Part model, mm, in its own coordinate system. A direction names the side the tool comes from. Coordinates: 2 decimals unless noted, no trailing zeros. Write each loop counter-clockwise with the first axis right and the second up, starting at its lowest first coordinate (ties: lowest second). Pieces come first, ordered by that corner, then holes. Notation, with made-up numbers: (61.25, 64.5) -> (89.25, 64.5) arc R15 cw to (89.25, 85.5) -> close; hole circle Ø9 at (44, 24.25). An arc over 180 degrees is marked (long way). One line per question, with ' | ' between items. Start each with the question number.
Item 1: Pin check, flat tips, straight feed: pin 1 (3.5 mm diameter, centred on x = 1.5, y = 0, fed in from -Z); pin 2 (4 mm diameter, centred on x = -12.5, y = 4, fed in from +Z); pin 3 (0.8 mm diameter, centred on x = 4, z = -1, fed in from +Y); pin 4 (2 mm diameter, centred on x = 7, z = 0.15, fed in from +Y). Stop position of each tip, or through.
Item 2: Saw through at D-D (z = 5). List the corners of the cut face in (x, y).
Item 3: Saw through at C-C (y = 0). Count the separate pieces of the cut face and the enclosed holes in it, and give its area (3 significant figures).
Item 4: Two-plate mould, pull along X, no slides. Class faces 1 (the flat face through (4, 1, -2)), 2 (the cylindrical face through (3, 0, 10)), 3 (the cylindrical face through (-17.32, -1.7, -11.74)), 4 (the cylindrical face through (5.29, 0.08, -0.23)): pulls with the +X half, pulls with the -X half, needs draft (parallel to the pull), parting line crosses it, or undercut.
Item 5: Probe probe 1 along Y at (x, z) = (-8, -6.35); probe 2 along Z at (x, y) = (3.5, 0.5); probe 3 along X at (y, z) = (-4, 1.25) (3 decimals). List the from-to ranges inside material, lowest first. Write a range as [from, to].
Item 6: Saw through at A-A (x = -7). List the corners of the cut face in (y, z), and give its area (3 significant figures).
Item 7: Saw through at B-B (x = 0). List the corners of the cut face in (y, z), and give its area (3 significant figures).
Item 8: 3-axis set-ups, long thin cutter, end or side, ignore diameter. For faces 5 (the cylindrical face through (7.751, -0.079, 2.535)), 6 (the cylindrical face through (-5.39, -1.7, 10.97)), 7 (the cylindrical face through (0, 2.5, -2)), 8 (the flat face through (4, -1, -2)): which of +Z, -Z, +X, -X, +Y, -Y reach the whole face in a straight line?
from build123d import *

# Parameters (mm, degrees)
BOSS_EXTRUDE1_DEPTH      = 5.65
BOSS_EXTRUDE1_DEPTH_BACK = 5.65
SKETCH6_R                = 2.5
SKETCH7_R                = 1.75
CUT_EXTRUDE1_DEPTH       = 22.626141761
BOSS_EXTRUDE3_DEPTH      = 1
BOSS_EXTRUDE3_DEPTH_BACK = 1
SKETCH8_W                = 10.3
SKETCH8_H                = 5
CHAMFER1_SIZE            = 0.5
SKETCH9_R                = 5.15
BOSS_EXTRUDE4_DEPTH      = 1.3333
BOSS_EXTRUDE5_START      = 1.3333
SKETCH10_R               = 5.15
BOSS_EXTRUDE5_DEPTH      = 1.3333
SKETCH11_R               = 5.15
BOSS_EXTRUDE6_DEPTH      = 1.333
SKETCH14_R               = 2
CUT_EXTRUDE2_DEPTH       = 39.36556716
CUT_EXTRUDE3_REACH       = 32.253
CUT_EXTRUDE3_END_RADIUS  = 2
SKETCH16_R               = 2


with BuildPart() as part:
    # Sketch4 → Revolve1 (revolve)
    with BuildSketch(Plane(origin=(0, 0, 0), x_dir=(1, 0, 0), z_dir=(0, 1, 0)), mode=Mode.PRIVATE) as revolve1_sk:
        Polygon((-14, 6.35), (-14, 12), (-5.5, 12), (-4, 9.85), (4, 9.85), (5.5, 12), (14, 12), (14, 6.35), align=None)
    revolve(revolve1_sk.sketch.rotate(Axis((-14, 0, -6.35), (1, 0, 0)), 180), axis=Axis((-14, 0, -6.35), (1, 0, 0)))

    # Sketch5 → Revolve2 (revolve)
    with BuildSketch(Plane(origin=(0, 0, 0), x_dir=(1, 0, 0), z_dir=(0, 1, 0)), mode=Mode.PRIVATE) as revolve2_sk:
        Polygon((-2.5, 2.85), (-2.5, 0.85), (-5.65, -0.65), (-5.65, -7.65), (0, -7.65), (0, 6.35), (-2.5, 6.35), align=None)
    revolve(revolve2_sk.sketch.rotate(Axis((0, 0, 7.65), (0, 0, -1)), 180), axis=Axis((0, 0, 7.65), (0, 0, -1)))

    # Sketch6 → Boss-Extrude1 (add, two sides: drawn at the far end of the back side and taken through both)
    with BuildSketch(Plane(origin=(0, 0, 0), x_dir=(1, 0, 0), z_dir=(0, 1, 0)).offset(-BOSS_EXTRUDE1_DEPTH_BACK)):
        with Locations(Location((-7, -0.15, 0), (0, 0, 270))):
            Circle(SKETCH6_R)
        with Locations(Location((7, -0.15, 0), (0, 0, 270))):
            Circle(SKETCH6_R)
    extrude(amount=BOSS_EXTRUDE1_DEPTH + BOSS_EXTRUDE1_DEPTH_BACK)

    # Sketch7 → Cut-Extrude1 (cut, through all)
    with BuildSketch(Plane(origin=(0, 5.65, 0), x_dir=(1, 0, 0), z_dir=(0, 1, 0))):
        with Locations(Location((7, -0.15, 0), (0, 0, 270))):
            Circle(SKETCH7_R)
        with Locations(Location((-7, -0.15, 0), (0, 0, 270))):
            Circle(SKETCH7_R)
    extrude(amount=-CUT_EXTRUDE1_DEPTH, mode=Mode.SUBTRACT)

    # Sketch8 → Boss-Extrude3 (add, two sides: drawn at the far end of the back side and taken through both)
    with BuildSketch(Plane(origin=(0, 0, 0), x_dir=(1, 0, 0), z_dir=(0, 1, 0)).offset(-BOSS_EXTRUDE3_DEPTH_BACK)):
        with Locations((0, 2)):
            Rectangle(SKETCH8_W, SKETCH8_H)
    extrude(amount=BOSS_EXTRUDE3_DEPTH + BOSS_EXTRUDE3_DEPTH_BACK)

    # Chamfer1
    chamfer1_edges = [part.edges().sort_by_distance(p)[0] for p in [
        (14, 0, -12),
        (-5.65, 0, 7.65),
        (-14, 0, -12),
    ]]
    chamfer(chamfer1_edges, length=CHAMFER1_SIZE)

    # Sketch9 → Boss-Extrude4 (add)
    with BuildSketch(Plane(origin=(14, 0, 0), x_dir=(0, 0, -1), z_dir=(1, 0, 0))):
        with Locations(Location((6.35, 0, 0), (0, 0, 180))):
            Circle(SKETCH9_R)
    extrude(amount=BOSS_EXTRUDE4_DEPTH)

    # Sketch10 → Boss-Extrude5 (add)
    with BuildSketch(Plane.ZY.offset(14).offset(BOSS_EXTRUDE5_START)):
        with Locations((-6.35, 0)):
            Circle(SKETCH10_R)
    extrude(amount=-BOSS_EXTRUDE5_DEPTH)

    # Sketch11 → Boss-Extrude6 (add)
    with BuildSketch(Plane.XY.offset(7.65)):
        with Locations(Location((0, 0, 0), (0, 0, 180))):
            Circle(SKETCH11_R)
    extrude(amount=BOSS_EXTRUDE6_DEPTH)

    # Sketch12 → Revolve3 (revolve)
    with BuildSketch(Plane(origin=(0, 0, 0), x_dir=(1, 0, 0), z_dir=(0, 1, 0))):
        Polygon((15.3333, 6.35), (17.99996, 6.35), (17.99996, 12), (16.66663, 12), (16.66663, 9.35), (15.3333, 9.35), align=None)
        Polygon((-16.66663, 9.35), (-15.3333, 9.35), (-15.3333, 6.35), (-17.99996, 6.35), (-17.99996, 12), (-16.66663, 12), align=None)
    revolve(axis=Axis((-15.3333, 0, -6.35), (-1, 0, 0)))

    # Sketch13 → Revolve4 (revolve)
    with BuildSketch(Plane(origin=(0, 0, 0), x_dir=(1, 0, 0), z_dir=(0, 1, 0))):
        Polygon((0, -8.983), (0, -11.64966), (-5.65, -11.64966), (-5.65, -10.31633), (-3, -10.31633), (-3, -8.983), align=None)
    revolve(axis=Axis((0, 0, 8.983), (0, 0, 1)))

    # Sketch14 → Cut-Extrude2 (cut, through all)
    with BuildSketch(Plane(origin=(17.99996, 0, 0), x_dir=(0, 0, -1), z_dir=(1, 0, 0))):
        with Locations((6.35, 0)):
            Circle(SKETCH14_R)
    extrude(amount=-CUT_EXTRUDE2_DEPTH, mode=Mode.SUBTRACT)

    # Cut-Extrude3: up to this cylinder (the profile starts outside it)
    cut_extrude3_end = Plane(origin=(0, 0, -6.35), z_dir=(1, 0, 0)) * Cylinder(CUT_EXTRUDE3_END_RADIUS, 69.506, mode=Mode.PRIVATE)
    # Sketch16 → Cut-Extrude3 (cut, up to the surface)
    with BuildSketch(Plane.XY.offset(11.64966), mode=Mode.PRIVATE) as cut_extrude3_sk1:
        Circle(SKETCH16_R)
    cut_extrude3_tool1 = extrude(cut_extrude3_sk1.sketch, amount=-CUT_EXTRUDE3_REACH, mode=Mode.PRIVATE) - cut_extrude3_end
    add(cut_extrude3_tool1.solids().sort_by_distance((0, 0, 11.64966))[0], mode=Mode.SUBTRACT)


solid = part.part
From the geometry:
1) pin 1: z = -9.85 | pin 2: z = -1.07 | pin 3: y = 1 | pin 4: through
2) outline: circle Ø11.3 at (0, 0); hole circle Ø4 at (0, 0)
3) separate pieces: 3 | enclosed holes: 2 | area: 295 mm2
4) face 1: undercut | face 2: parting line crosses it | face 3: needs draft | face 4: undercut
5) probe 1: [-5.65, -2], [2, 5.65] | probe 2: [-9.81, -8.29], [-4.41, 8.98], [10.32, 11.65] | probe 3: [-9.245, -8.361], [-5.639, -4.755], [-3.99, 3.99], [4.755, 5.639], [8.361, 9.245]
6) outline: (-5.65, -2.35) -> (-3.99, -2.35) arc R5.65 ccw (long way) to (3.99, -2.35) -> (5.65, -2.35) -> (5.65, -1.6) -> (-5.65, -1.6) -> close; (-5.65, 1.9) -> (5.65, 1.9) -> (5.65, 2.65) -> (-5.65, 2.65) -> close; hole circle Ø4 at (0, -6.35) | area: 95.6 mm2
7) outline: (-5.65, 0.65) -> (-2.5, -0.85) -> (-2.5, -3.9) arc R3.5 ccw (long way) to (2.5, -3.9) -> (2.5, -0.85) -> (5.65, 0.65) -> (5.65, 7.15) -> (5.15, 7.65) -> (5.15, 8.98) -> (3, 8.98) -> (3, 10.32) -> (5.65, 10.32) -> (5.65, 11.65) -> (2, 11.65) -> (2, -6.35) arc R2 cw to (-2, -6.35) -> (-2, 11.65) -> (-5.65, 11.65) -> (-5.65, 10.32) -> (-3, 10.32) -> (-3, 8.98) -> (-5.15, 8.98) -> (-5.15, 7.65) -> (-5.65, 7.15) -> close | area: 99.7 mm2
8) face 5: none | face 6: +Z | face 7: +Y | face 8: -Y
